```python
from build123d import *

# Parameters (mm, degrees)
SKIZZE1_W                                    = 50
SKIZZE1_H                                    = 50
AUFSATZ_LINEAR_AUSTRAGEN1_DEPTH              = 40
SKIZZE2_W                                    = 12.5
SKIZZE2_H                                    = 50
SKIZZE2_W_2                                  = 25
SCHNITT_LINEAR_AUSTRAGEN1_DEPTH              = 30
STIRNSENKUNG_F_R_M4_FLACHKOPFSCHRAUB_2_COUNT = 2
STIRNSENKUNG_F_R_M4_FLACHKOPFSCHRAUB_2_PITCH = 36
STIRNSENKUNG_F_R_M4_FLACHKOPFSCHRAUB_3_COUNT = 2
STIRNSENKUNG_F_R_M4_FLACHKOPFSCHRAUB_3_PITCH = 36
STIRNSENKUNG_F_R_M4_FLACHKOPFSCHRAUB_4_COUNT = 2
STIRNSENKUNG_F_R_M4_FLACHKOPFSCHRAUB_4_PITCH = 50.911688245
VERST_RKUNGSRIPPE4_REACH                     = 55.385
SKIZZE7_WALL_W                               = 147.8220309
SKIZZE7_WALL_H                               = 8
VERRUNDUNG1_R                                = 4
DURCHGANGSLOCH_F_R_M41_D                     = 4.5
F_3_0_3_DURCHMESSER_BOHRUNG1_D               = 3
M4_GEWINDEBOHRUNG1_AT_2_COUNT                = 2
M4_GEWINDEBOHRUNG1_AT_2_PITCH                = 12


with BuildPart() as part:
    # Skizze1 → Aufsatz-Linear austragen1 (new body)
    with BuildSketch(Plane(origin=(0, 0, 0), x_dir=(1, 0, 0), z_dir=(0, 1, 0))):
        Rectangle(SKIZZE1_W, SKIZZE1_H)
    extrude(amount=AUFSATZ_LINEAR_AUSTRAGEN1_DEPTH)

    # Skizze2 → Schnitt-Linear austragen1 (cut)
    with BuildSketch(Plane(origin=(0, 40, 0), x_dir=(1, 0, 0), z_dir=(0, 1, 0))):
        with Locations((-18.75, 0)):
            Rectangle(SKIZZE2_W, SKIZZE2_H)
        with Locations((12.5, 0)):
            Rectangle(SKIZZE2_W_2, SKIZZE2_H)
    extrude(amount=-SCHNITT_LINEAR_AUSTRAGEN1_DEPTH, mode=Mode.SUBTRACT)

    # Skizze4 → Stirnsenkung für M4 Flachkopfschraube mit Schlitz1 (revolve, cut)
    with BuildSketch(Plane(origin=(-18, 10, 18), x_dir=(0, 0, 1), z_dir=(1, 0, 0))):
        Polygon((0, 0), (0, 10), (2.25, 10), (2.25, 3.1), (4.5, 3.1), (4.5, 0.2), (4.7, 0), align=None)
    stirnsenkung_f_r_m4_flachkopfschraube_mi = revolve(axis=Axis((-18, 16.35, 18), (0, -1, 0)), mode=Mode.SUBTRACT)

    # Stirnsenkung f_r M4 Flachkopfschraub 2: Stirnsenkung für M4 Flachkopfschraube mit Schlitz1 ×2
    with Locations(*[(0, 0, -i * STIRNSENKUNG_F_R_M4_FLACHKOPFSCHRAUB_2_PITCH) for i in range(1, STIRNSENKUNG_F_R_M4_FLACHKOPFSCHRAUB_2_COUNT)]):
        add(stirnsenkung_f_r_m4_flachkopfschraube_mi, mode=Mode.SUBTRACT)

    # Stirnsenkung f_r M4 Flachkopfschraub 3: Stirnsenkung für M4 Flachkopfschraube mit Schlitz1 ×2
    with Locations(*[(i * STIRNSENKUNG_F_R_M4_FLACHKOPFSCHRAUB_3_PITCH, 0, 0) for i in range(1, STIRNSENKUNG_F_R_M4_FLACHKOPFSCHRAUB_3_COUNT)]):
        add(stirnsenkung_f_r_m4_flachkopfschraube_mi, mode=Mode.SUBTRACT)

    # Stirnsenkung f_r M4 Flachkopfschraub 4: Stirnsenkung für M4 Flachkopfschraube mit Schlitz1 ×2
    with Locations(*[Vector(0.7071067811865476, 0, -0.7071067811865476) * (i * STIRNSENKUNG_F_R_M4_FLACHKOPFSCHRAUB_4_PITCH) for i in range(1, STIRNSENKUNG_F_R_M4_FLACHKOPFSCHRAUB_4_COUNT)]):
        add(stirnsenkung_f_r_m4_flachkopfschraube_mi, mode=Mode.SUBTRACT)

    # Skizze7 wall → Verstärkungsrippe4 (add, up to next)
    with BuildSketch(Plane(origin=(12.5, 25, 0), x_dir=(0.640184399664, -0.768221279597, 0), z_dir=(0.768221279597, 0.640184399664, 0)), mode=Mode.PRIVATE) as verst_rkungsrippe4_sk1:
        Rectangle(SKIZZE7_WALL_W, SKIZZE7_WALL_H)
    verst_rkungsrippe4_tool1 = extrude(verst_rkungsrippe4_sk1.sketch, amount=-VERST_RKUNGSRIPPE4_REACH, mode=Mode.PRIVATE) - part.part
    add(verst_rkungsrippe4_tool1.solids().sort_by_distance((12.5, 25, 0))[0])

    # Verrundung1
    verrundung1_edges = [part.edges().sort_by_distance(p)[0] for p in [
        (0, 10, -14.5),
        (0, 10, 14.5),
        (12.5, 10, -4),
        (12.5, 10, 4),
        (0, 25, 4),
        (0, 25, -4),
    ]]
    fillet(verrundung1_edges, radius=VERRUNDUNG1_R)

    # Durchgangsloch für M41 (through all)
    with Locations(Plane(origin=(0, 0, 0), x_dir=(0, 0, -1), z_dir=(1, 0, 0))):
        with Locations((-18, 30), (18, 30)):
            Hole(DURCHGANGSLOCH_F_R_M41_D / 2)

    # Ø3.0 (3) Durchmesser Bohrung1 (through all)
    with Locations(Plane.ZY.offset(12.5)):
        with Locations((-10, 30), (10, 30)):
            Hole(F_3_0_3_DURCHMESSER_BOHRUNG1_D / 2)

    # Skizze14 → M4 Gewindebohrung1 (revolve, cut)
    with BuildSketch(Plane(origin=(-5, 35, -25), x_dir=(0, 1, 0), z_dir=(1, 0, 0))):
        Polygon((0, 0), (0, 12.491420021), (1.65, 11.5), (1.65, 0), align=None)
    m4_gewindebohrung1 = revolve(axis=Axis((-5, 35, -31.35), (0, 0, 1)), mode=Mode.SUBTRACT)

    # M4 Gewindebohrung1 at 2: M4 Gewindebohrung1 ×2
    with Locations(*[(0, -i * M4_GEWINDEBOHRUNG1_AT_2_PITCH, 0) for i in range(1, M4_GEWINDEBOHRUNG1_AT_2_COUNT)]):
        add(m4_gewindebohrung1, mode=Mode.SUBTRACT)

    # Spiegeln1: M4 Gewindebohrung1 across plane
    add(m4_gewindebohrung1.mirror(Plane.XY), mode=Mode.SUBTRACT)

    # Spiegeln1 copy 1 sketch → Spiegeln1 copy 1 (revolve, cut)
    with BuildSketch(Plane(origin=(-5, 23, 25), x_dir=(0, 1, 0), z_dir=(1, 0, 0))):
        Polygon((0, 0), (0, -12.491420021), (1.65, -11.5), (1.65, 0), align=None)
    revolve(axis=Axis((-5, 23, 31.35), (0, 0, 1)), mode=Mode.SUBTRACT)


solid = part.part
```
The listing builds one solid part. Answer for the finished solid, in the listing's coordinates (mm). A direction names the side the tool comes from. Give positions to 0.01 mm unless a question says otherwise; leave off trailing zeros. Write each loop counter-clockwise with the first axis right and the second up, starting at its lowest first coordinate (ties: lowest second). Pieces come first, ordered by that corner, then holes. Notation, with made-up numbers: (44.5, 25) - (49.5, 25) arc R25 ccw to (49.5, 38) - close; hole circle Ø7 at (-23.75, -9). An arc over 180 degrees is marked (long way). Use one line per item in the form item = value. Start each with the question number.
1) Flat-ended cylindrical pins translate along their axes: pin 1 Ø19.5 at (x, y) = (17, 26) entering from +Z; pin 2 Ø3 at (y, z) = (31.5, 10) entering from -X; pin 3 Ø2.5 at (x, z) = (-18, 18) entering from -Y; pin 4 Ø2 at (x, z) = (2.5, 18.5) entering from +Y. Find the tip coordinate at first contact, or state that the pin passes through.
2) Find section A-A on x = -18. Determine the outline of the cut face in (y, z), plus the area to 3 significant figures.
3) Consider line 1 along Y through (x, z) = (-5, 18); line 2 along X through (y, z) = (9, 18); line 3 along X through (y, z) = (1.5, 18). Determine where each line is inside the solid, lowest interval first. Write a range as from..to.
4) Find section D-D on x = -11.5. Determine the outline of the cut face in (y, z), plus the area to 3 significant figures.
5) A tool of negligible diameter and unlimited length cuts with its end or side. For faces 1 (the face through (22.39, 8.37, -18.98)), 2 (the face through (12, 10, 16)), 3 (the face through (9, 21, -4)), 4 (the face through (-12.5, 25, 0)), from which of +Z, -Z, +X, -X, +Y, -Y can it reach the whole face along a straight path? Write none if from no direction.
6) Find section C-C on y = 3.5. Determine the outline of the cut face in (x, z).
7) Find section B-B on z = -10. Determine the outline of the cut face in (x, y), plus the area to 3 significant figures.
8) The mould has two halves that part along Y. Classify faces 5 (the face through (-4.9, 23.3, 12.7)), 6 (the face through (14.353, 11.141, 5.203)), 7 (the face through (0, 27, -16)), 8 (the face through (0, 0, 0)): pulls with the +Y half, pulls with the -Y half, needs draft (parallel to the pull), parting line crosses it, or undercut.
Geometry results:
q1.pin_1 = 4
q1.pin_2 = -12.5
q1.pin_3 = through
q1.pin_4 = 10.88
q2.outline = (0, -25) - (10, -25) - (10, -22.7) - (9.8, -22.5) - (6.9, -22.5) - (6.9, -20.25) - (0, -20.25) - close; (0, -15.75) - (6.9, -15.75) - (6.9, -13.5) - (9.8, -13.5) - (10, -13.3) - (10, 13.3) - (9.8, 13.5) - (6.9, 13.5) - (6.9, 15.75) - (0, 15.75) - close; (0, 20.25) - (6.9, 20.25) - (6.9, 22.5) - (9.8, 22.5) - (10, 22.7) - (10, 25) - (0, 25) - close
q2.area = 382 mm2
q3.line_1 = 0..21.35, 24.65..27.75, 32.25..33.35, 36.65..40
q3.line_2 = -25..-22.5, -13.5..13.5, 22.5..25
q3.line_3 = -25..-20.25, -15.75..15.75, 20.25..25
q4.outline = (0, -25) - (40, -25) - (40, 25) - (0, 25) - close; hole circle Ø4.5 at (30, -18); hole circle Ø4.5 at (30, 18); hole circle Ø3 at (30, -10); hole circle Ø3 at (30, 10)
q4.area = 1,950 mm2
q5.face_1 = +Y
q5.face_2 = +Z, +X, +Y
q5.face_3 = -Z, +X, +Y
q5.face_4 = +Z, -Z, -X, +Y
q6.outline = (-25, -25) - (25, -25) - (25, 25) - (-25, 25) - close; hole circle Ø4.5 at (-18, -18); hole circle Ø4.5 at (-18, 18); hole circle Ø4.5 at (18, -18); hole circle Ø4.5 at (18, 18)
q7.outline = (-25, 0) - (25, 0) - (25, 10) - (4, 10) arc R4 cw to (0, 14) - (0, 28.5) - (-12.5, 28.5) - (-12.5, 10) - (-25, 10) - close; (-12.5, 31.5) - (0, 31.5) - (0, 40) - (-12.5, 40) - close
q7.area = 841 mm2
q8.face_5 = undercut
q8.face_6 = pulls with the +Y half
q8.face_7 = needs draft
q8.face_8 = pulls with the -Y half
